The drawing under review shows one solid part. Ordinate dimensions are in mm from its lowest x, y, z. Coordinates: 2 decimals unless noted, no trailing zeros. Order: outer loops, then holes, each group sorted by start corner. A loop starts at its lowest first (then second) coordinate and runs counter-clockwise, first axis right, second up.
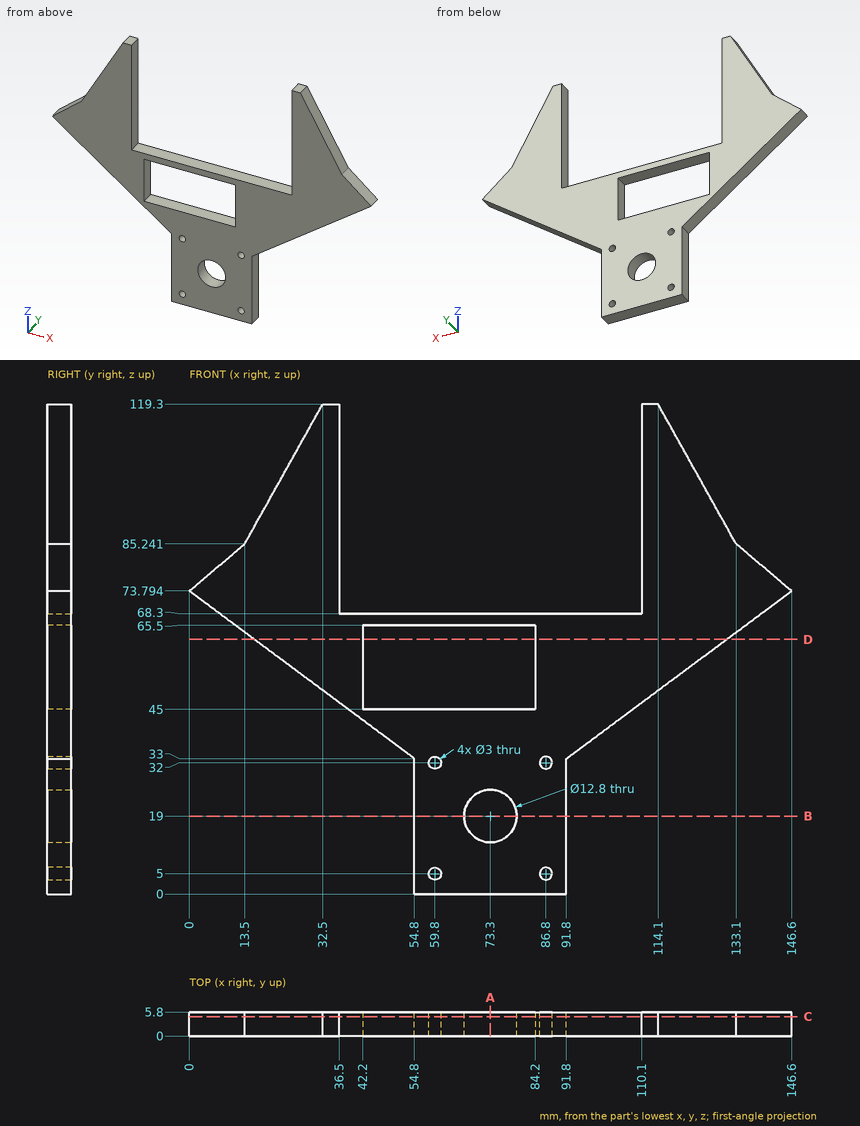
(1) We need section A-A, the plane x = 73.3. Write out the cut boundary in (y, z).
A:
outline: (0, 0) - (5.8, 0) - (5.8, 12.6) - (0, 12.6) - close; (0, 25.4) - (5.8, 25.4) - (5.8, 45) - (0, 45) - close; (0, 65.5) - (5.8, 65.5) - (5.8, 68.3) - (0, 68.3) - close
(2) Wall thickness on probe 1 along X at (y, z) = (3.15, 32); probe 2 along Z at (x, y) = (59.8, 4.05); probe 3 along Z at (x, y) = (86.8, 2.3): over which ranges is each line inside the solid? List them lowest first.
A:
probe 1: x = 54.8 to 58.3, 61.3 to 85.3, 88.3 to 91.8
probe 2: z = 0 to 3.5, 6.5 to 30.5, 33.5 to 45, 65.5 to 68.3
probe 3: z = 0 to 3.5, 6.5 to 30.5, 33.5 to 68.3
(3) For pin 1 Ø1.7 at (y, z) = (2, 9.5) entering from -X; pin 2 Ø1.5 at (x, y) = (41, 2) entering from -Z (1 decimal); pin 3 Ø1.7 at (y, z) = (3.5, 15.5) entering from +X, all flat-tipped, find the tip position at first contact; note any pin that passes through.
A:
pin 1: stops at x = 54.8
pin 2: stops at z = 42.7
pin 3: stops at x = 91.8
(4) We need section D-D, the plane z = 62. Write out the cut boundary in (x, y), and give its area (3 significant figures).
A:
outline: (15.84, 0) - (42.2, 0) - (42.2, 5.8) - (15.84, 5.8) - close; (84.2, 0) - (130.76, 0) - (130.76, 5.8) - (84.2, 5.8) - close
area: 423 mm2
(5) We need section C-C, the plane y = 4.7. Write out the cut boundary in (x, z).
A:
outline: (0, 73.79) - (54.8, 33) - (54.8, 0) - (91.8, 0) - (91.8, 33) - (146.6, 73.79) - (133.1, 85.24) - (114.1, 119.3) - (110.1, 119.3) - (110.1, 68.3) - (36.5, 68.3) - (36.5, 119.3) - (32.5, 119.3) - (13.5, 85.24) - close; hole (42.2, 45) - (84.2, 45) - (84.2, 65.5) - (42.2, 65.5) - close; hole circle Ø3 at (59.8, 5); hole circle Ø3 at (59.8, 32); hole circle Ø12.8 at (73.3, 19); hole circle Ø3 at (86.8, 5); hole circle Ø3 at (86.8, 32)
(6) We need section B-B, the plane z = 19. Write out the cut boundary in (x, y), and give its area (3 significant figures).
A:
outline: (54.8, 0) - (66.9, 0) - (66.9, 5.8) - (54.8, 5.8) - close; (79.7, 0) - (91.8, 0) - (91.8, 5.8) - (79.7, 5.8) - close
area: 140 mm2
